```python
from build123d import *

# Parameters (mm, degrees)
SKETCH4_W               = 84.5
SKETCH4_H               = 84
BOSS_EXTRUDE1_DEPTH     = 8.175
SKETCH5_W               = 84.5
SKETCH5_H               = 5
BOSS_EXTRUDE2_DEPTH     = 48
SKETCH6_R               = 2.225
CUT_EXTRUDE1_DEPTH      = 48
SKETCH7_W               = 7.5
SKETCH7_H               = 84
BOSS_EXTRUDE3_DEPTH     = 31.675
SKETCH8_W               = 2.5
SKETCH8_H               = 84
BOSS_EXTRUDE4_DEPTH     = 11.5
CUT_EXTRUDE2_DEPTH      = 93
CUT_EXTRUDE2_DEPTH_BACK = 5
SKETCH9_R               = 3
SKETCH10_W              = 7.5
SKETCH10_H              = 84
BOSS_EXTRUDE5_DEPTH     = 2.5
FILLET1_R               = 1
CUT_EXTRUDE3_DEPTH      = 88
CUT_EXTRUDE3_DEPTH_BACK = 24.5
FILLET2_R               = 10
FILLET3_R               = 5
FILLET4_R               = 15.75


with BuildPart() as part:
    # Sketch4 → Boss-Extrude1 (new body)
    with BuildSketch(Plane(origin=(0, 25, 0), x_dir=(1, 0, 0), z_dir=(0, 1, 0))):
        with Locations((10, 37)):
            Rectangle(SKETCH4_W, SKETCH4_H)
    extrude(amount=BOSS_EXTRUDE1_DEPTH)

    # Sketch5 → Boss-Extrude2 (add)
    with BuildSketch(Plane.XZ.offset(-25)):
        with Locations((10, 2.5)):
            Rectangle(SKETCH5_W, SKETCH5_H)
        with Locations((10, -76.5)):
            Rectangle(SKETCH5_W, SKETCH5_H)
    extrude(amount=BOSS_EXTRUDE2_DEPTH)

    # Sketch6 → Cut-Extrude1 (cut)
    with BuildSketch(Plane.XZ.offset(-25)):
        with Locations(Location((-1, -21, 0), (0, 0, 270))):
            Circle(SKETCH6_R)
        with Locations(Location((-1, -53, 0), (0, 0, 270))):
            Circle(SKETCH6_R)
    extrude(amount=-CUT_EXTRUDE1_DEPTH, mode=Mode.SUBTRACT)

    # Sketch7 → Boss-Extrude3 (add)
    with BuildSketch(Plane(origin=(0, 33.175, 0), x_dir=(1, 0, 0), z_dir=(0, 1, 0))):
        with Locations((-28.5, 37)):
            Rectangle(SKETCH7_W, SKETCH7_H)
        with Locations((48.5, 37)):
            Rectangle(SKETCH7_W, SKETCH7_H)
    extrude(amount=BOSS_EXTRUDE3_DEPTH)

    # Sketch8 → Boss-Extrude4 (add)
    with BuildSketch(Plane(origin=(0, 64.85, 0), x_dir=(1, 0, 0), z_dir=(0, 1, 0))):
        with Locations((-31, 37)):
            Rectangle(SKETCH8_W, SKETCH8_H)
        with Locations((51, 37)):
            Rectangle(SKETCH8_W, SKETCH8_H)
    extrude(amount=BOSS_EXTRUDE4_DEPTH)

    # Sketch9 → Cut-Extrude2 (cut, two sides: drawn at the far end of the back side and taken through both)
    with BuildSketch(Plane(origin=(0, 0, 0), x_dir=(-1, 0, 0), z_dir=(0, 0, -1)).offset(-CUT_EXTRUDE2_DEPTH_BACK)):
        with Locations(Location((-10, -17, 0), (0, 0, 270))):
            Circle(SKETCH9_R)
        with Locations(Location((-24.5, -17, 0), (0, 0, 270))):
            Circle(SKETCH9_R)
        with Locations(Location((4.5, -17, 0), (0, 0, 270))):
            Circle(SKETCH9_R)
    extrude(amount=CUT_EXTRUDE2_DEPTH + CUT_EXTRUDE2_DEPTH_BACK, mode=Mode.SUBTRACT)

    # Sketch10 → Boss-Extrude5 (add)
    with BuildSketch(Plane(origin=(0, 76.35, 0), x_dir=(1, 0, 0), z_dir=(0, 1, 0))):
        with Locations((48.5, 37)):
            Rectangle(SKETCH10_W, SKETCH10_H)
        with Locations((-28.5, 37)):
            Rectangle(SKETCH10_W, SKETCH10_H)
    extrude(amount=BOSS_EXTRUDE5_DEPTH)

    # Fillet1
    fillet1_edges = [part.edges().sort_by_distance(p)[0] for p in [
        (47.25, 76.35, -79),
        (44.75, 76.35, -37),
        (47.25, 76.35, 5),
        (52.25, 78.85, -37),
        (48.5, 78.85, -79),
        (44.75, 78.85, -37),
        (48.5, 78.85, 5),
        (-27.25, 76.35, 5),
        (-24.75, 76.35, -37),
        (-27.25, 76.35, -79),
        (-32.25, 78.85, -37),
        (-28.5, 78.85, 5),
        (-24.75, 78.85, -37),
        (-28.5, 78.85, -79),
        (-24.75, 64.85, -37),
        (-27.25, 64.85, -79),
        (44.75, 64.85, -37),
        (47.25, 64.85, 5),
        (-27.25, 64.85, 5),
        (47.25, 64.85, -79),
        (-29.75, 64.85, -37),
        (-29.75, 70.6, 5),
        (-29.75, 70.6, -79),
        (-29.75, 76.35, -37),
        (49.75, 64.85, -37),
        (49.75, 70.6, -79),
        (49.75, 70.6, 5),
        (49.75, 76.35, -37),
    ]]
    fillet(fillet1_edges, radius=FILLET1_R)

    # Sketch11 → Cut-Extrude3 (cut, two sides: drawn at the far end of the back side and taken through both)
    with BuildSketch(Plane(origin=(0, 0, 0), x_dir=(-1, 0, 0), z_dir=(0, 0, -1)).offset(-CUT_EXTRUDE3_DEPTH_BACK)):
        Polygon((19, -23), (32.25, -23), (32.25, 25), align=None)
        Polygon((-39, -23), (-52.25, -23), (-52.25, 25), align=None)
    extrude(amount=CUT_EXTRUDE3_DEPTH + CUT_EXTRUDE3_DEPTH_BACK, mode=Mode.SUBTRACT)

    # Fillet2
    fillet2_edges = [part.edges().sort_by_distance(p)[0] for p in [
        (39, -23, 2.5),
        (-19, -23, 2.5),
        (-19, -23, -76.5),
        (39, -23, -76.5),
    ]]
    fillet(fillet2_edges, radius=FILLET2_R)

    # Fillet3
    fillet3_edges = [part.edges().sort_by_distance(p)[0] for p in [
        (-24.75, 33.175, -37),
        (44.75, 33.175, -37),
    ]]
    fillet(fillet3_edges, radius=FILLET3_R)

    # Fillet4
    fillet4_edges = [part.edges().sort_by_distance(p)[0] for p in [
        (10, 25, 0),
        (10, 25, -74),
    ]]
    fillet(fillet4_edges, radius=FILLET4_R)


solid = part.part
```
Work out the finished part from the listing and answer in its coordinate system (mm). A direction names the side the tool comes from. Round coordinates to 2 decimals unless told otherwise and drop trailing zeros. Loops run counter-clockwise (first coordinate to the right, second up) from the corner with the lowest first, then second, coordinate; pieces in that order, holes last. Notation, with made-up numbers: M 49.5,87.25 L 91.5,87.25 A22 ccw 91.5,99.25 Z; hole C 35,-28.5 d10. An arc over 180 degrees is marked long. Use CSV: the item, a comma, the result in double quotes.
Q1. The mould has two halves that part along Z. Classify faces 4 (the flat face through (9, -7, 0)), 5 (the flat face through (52.25, 51, -36)), 6 (the flat face through (9, 16, 5)), 7 (the flat face through (9, 25, -37)): pulls with the +Z half, pulls with the -Z half, needs draft (parallel to the pull), parting line crosses it, or undercut.
Determined:
face 4,"undercut"
face 5,"needs draft"
face 6,"pulls with the +Z half"
face 7,"undercut"
Q2. Section B-B, the plane y = 47 is taken. Determine the outline of the cut face in (x, z), then the cut area to 3 significant figures.
Determined:
outline,"M -32.25,-79 L -24.75,-79 L -24.75,5 L -32.25,5 Z; M 44.75,-79 L 52.25,-79 L 52.25,5 L 44.75,5 Z"
area,"1,260 mm2"
Q3. Consider L1, parallel to Z at x = 25, y = 9; L2, parallel to Y at x = 24.5, z = 1.2 (3 decimals); L3, parallel to X at y = -17, z = -77. Determine where each line is inside the solid, lowest interval first.
Determined:
L1,"-79 to -74, 0 to 5"
L2,"-23 to -20, -14 to 33.175"
L3,"-20.55 to -7.5, -1.5 to 7, 13 to 21.5, 27.5 to 40.55"
Q4. Section C-C, the plane x = -4.5 is taken. Determine the outline of the cut face in (y, z) (3 decimals), then the cut area to 3 significant figures.
Determined:
outline,"M -23,-79 L -20,-79 L -20,-74 L -23,-74 Z; M -23,0 L -20,0 L -20,5 L -23,5 Z; M -14,-79 L 33.175,-79 L 33.175,5 L -14,5 L -14,0 L 9.25,0 A15.75 cw 25,-15.75 L 25,-58.25 A15.75 cw 9.25,-74 L -14,-74 Z"
area,"1,210 mm2"
Q5. A tool of negligible diameter and unlimited length cuts with its end or side. For faces 1 (the flat face through (10, -23, -76)), 2 (the flat face through (-29.75, 71, -36)), 3 (the cylindrical face through (43.246, 34.601, -37.588)), from which of +Z, -Z, +X, -X, +Y, -Y can it reach the whole face along a straight path? Write none if from no direction.
Determined:
face 1,"+Z, -Z, +X, -X, -Y"
face 2,"+Z, -Z"
face 3,"+Z, -Z, +Y"
Q6. Each of these flat-tipped pins is pushed along its axis until it touches: pin 1 (2 mm diameter, centred on x = -17.5, z = -48, fed in from +Y) (3 decimals); pin 2 (2.5 mm diameter, centred on x = 47.5, z = -41.5, fed in from -Y); pin 3 (4 mm diameter, centred on x = -23.5, z = -48, fed in from +Y). Where does it stop, or does it pass through?
Determined:
pin 1,"y = 33.175"
pin 2,"y = 25"
pin 3,"y = 78.82"
